Answer from the drawing. Dimensions are ordinates in mm from the lowest x, y and z of the part. Round coordinates to 2 decimals unless told otherwise and drop trailing zeros. Order: outer loops, then holes, each group sorted by start corner. A loop starts at its lowest first (then second) coordinate and runs counter-clockwise, first axis right, second up. Notation, with made-up numbers: M -12.5,64.5 L -6.5,64.5 A19 cw -6.5,92.5 Z; hole C 2.5,79.25 d11. An arc over 180 degrees is marked long. Use one line per item in the form item = value. Start each with the question number.
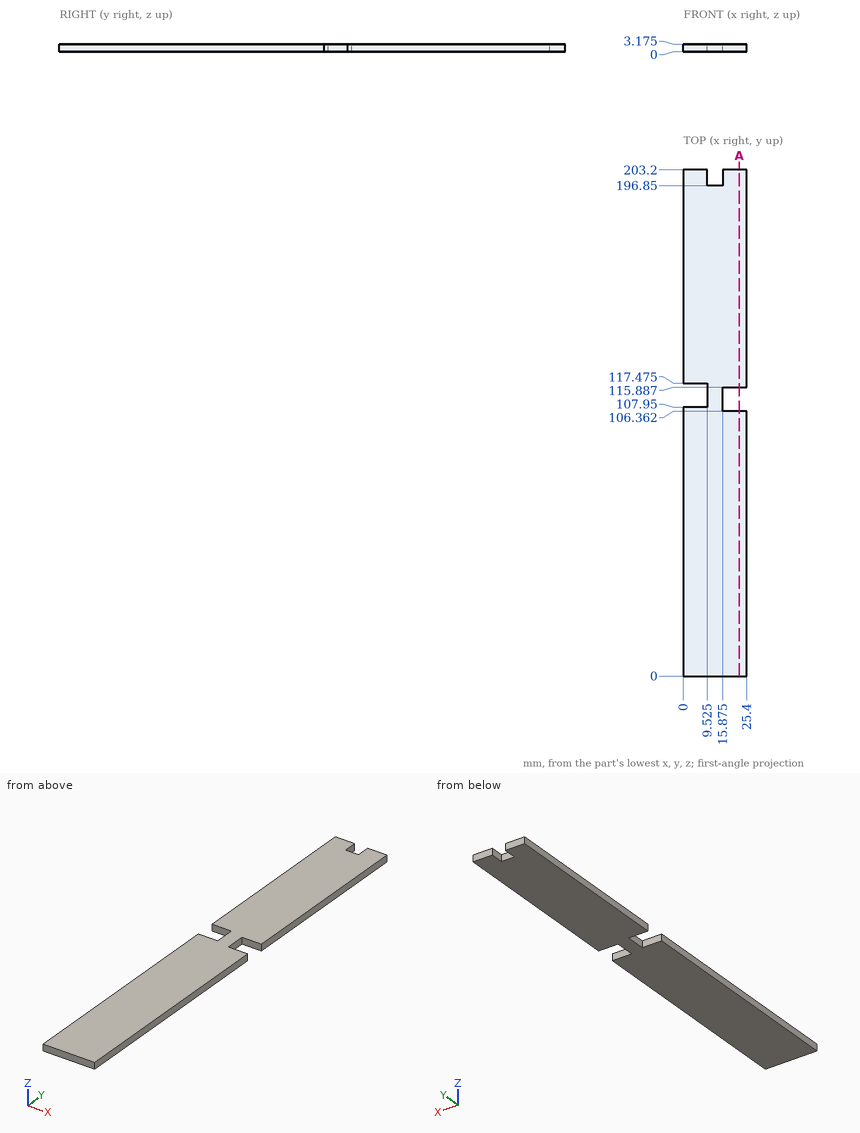
Item 1: Section A-A (x = 22.5) is taken. Write down the section's boundary in (y, z) (1 decimal), and give its area (3 significant figures).
Item 2: Find the intervals of material crossed by L1, parallel to Y at x = 21.5, z = 0.45; L2, parallel to X at y = 116, z = 0.4 (1 decimal); L3, parallel to Y at x = 12, z = 1, in increasing order. Write a range as [from, to].
Item 3: Given P1, Ø1.6, axis at y = 114, z = 1.5, coming from the -X side (1 decimal), flat-ended and moving along its own axis, determine where the tip first touches the part or whether it passes through.
The answers:
q1.outline = M 0,0 L 106.4,0 L 106.4,3.2 L 0,3.2 Z; M 115.9,0 L 203.2,0 L 203.2,3.2 L 115.9,3.2 Z
q1.area = 615 mm²
q2.L1 = [0, 106.36], [115.89, 203.2]
q2.L2 = [9.5, 25.4]
q2.L3 = [0, 196.85]
q3.P1 = 9.5
